The listing builds one solid part. Answer for the finished solid, in the listing's coordinates (mm). A direction names the side the tool comes from. Give positions to 0.01 mm unless a question says otherwise; leave off trailing zeros. Loops run counter-clockwise (first coordinate to the right, second up) from the corner with the lowest first, then second, coordinate; pieces in that order, holes last.
Item 1: Section D-D, the plane y = 31 is taken. Give the vertices of the cut face in (x, z), and give its area (3 significant figures).
Item 2: Section B-B, the plane x = -30 is taken. Give the vertices of the cut face in (y, z).
Item 3: The mould has two halves that part along Z. Classify faces 3 (the face through (75.507, 15.2, 9.693)), 4 (the face through (-1.064, -6.702, 3.125)), 5 (the face through (-76, 15, 20)), 6 (the face through (-60.073, -7.059, 27.407)): pulls with the +Z half, pulls with the -Z half, needs draft (parallel to the pull), parting line crosses it, or undercut.
Item 4: A tool of negligible diameter and unlimited length cuts with its end or side. For faces 1 (the face through (-75.493, 15.2, 9.693)), 2 (the face through (75, 15, 20)), from which of +Z, -Z, +X, -X, +Y, -Y can it reach the whole face along a straight path? Write none if from no direction.
Item 5: Section C-C, the plane y = -3.5 is taken. Give the vertices of the cut face in (x, z).
Item 6: Consider line 1 along X through (y, z) = (30, 21.5); line 2 along Z through (x, y) = (39, 1.5); line 3 along Z through (x, y) = (-33.5, 26). Determine where each line is inside the solid, lowest interval first.
Item 7: Each of these flat-tipped pins is pushed along its axis until it touches: pin 1 Ø12 at (x, z) = (-32.5, 35) entering from -Y; pin 2 Ø1.5 at (x, z) = (-46, 11) entering from -Y; pin 3 Ø6 at (x, z) = (-40, 41.5) entering from +Y. Where does it stop, or does it pass through?
Item 8: Section A-A, the plane y = 8 is taken. Give the vertices of the cut face in (x, z), and give its area (3 significant figures).
Autodesk Fusion 360 part; units mm, degrees
sketch "Sketch1" plane through (0, 0, 0) normal (1, 0, 0) x (0, 1, 0)
  line L0 (0, 0) -> (60, 0)
  line L1 (60, 0) -> (49.9725, 11.9503)
  line L2 (49.9725, 11.9503) -> (9.9318, 49.9475)
  line L3 (49.9725, 11.9503) -> (105.1725, 11.9503) construction
  line L4 (9.9318, 49.9475) -> (-0.0682, 49.9475)
  line L5 (0, 0) -> (-13.5946, 6.3393)
  line L6 (0, 0) -> (15, 0) construction
  line L7 (-13.5946, 6.3393) -> (-0.0682, 49.9475)
  dimension "d15" = 60
  dimension "d16" = 15.6
  dimension "d18" = 136.5
  dimension "d19" = 55.2
  dimension "d24" = 155
  dimension "d25" = 15
extrude "Extrude1" add sketch "Sketch1" along normal mid plane 152
shell "Shell1" thickness 1 removed faces 2 at (25.3333, 23.2787, 37.2817) at (25.3333, 56.6575, 3.9834)
sketch "Sketch3" plane through (0, -14.1952, 4.4031) normal (0, -0.9551, 0.2963) x (1, 0, 0)
  line L0 (-76, 2.0272) -> (76, 2.0272)
  line L1 (76, 2.0272) -> (76, 47.685)
  line L2 (76, 47.685) -> (-76, 47.685)
  line L3 (-76, 47.685) -> (-76, 2.0272)
  line L4 (0, 2.0272) -> (0, 47.685)
  line L5 (-69, 24.0272) -> (-69, 33.0272)
  line L6 (-69, 24.0272) -> (-69, 15.0272)
  line L7 (-69, 33.0272) -> (-51, 33.0272)
  line L8 (-51, 33.0272) -> (-51, 15.0272)
  line L9 (-51, 15.0272) -> (-69, 15.0272)
  line L10 (69, 33.0272) -> (51, 33.0272)
  line L11 (51, 33.0272) -> (51, 15.0272)
  line L12 (51, 15.0272) -> (69, 15.0272)
  line L13 (69, 24.0272) -> (69, 15.0272)
  line L14 (69, 24.0272) -> (69, 33.0272)
extrude "Extrude3" add sketch "Sketch3" along normal blind 28 contours L5 L6 L7 L8 L9 | L10 L11 L12 L13 L14
sketch "Sketch4" plane through (0, -40.9382, 12.6983) normal (0, -0.9551, 0.2963) x (1, 0, 0)
  line L0 (-69, 33.0272) -> (-69, 15.0272)
  line L1 (-69, 15.0272) -> (-51, 15.0272)
  line L2 (-51, 15.0272) -> (-51, 33.0272)
  line L3 (-51, 33.0272) -> (-69, 33.0272)
  line L4 (-54.8, 30.2) -> (-65.2, 30.2)
  line L5 (-65.2, 30.2) -> (-65.2, 17.8)
  line L6 (-65.2, 17.8) -> (-54.8, 17.8)
  line L7 (-54.8, 17.8) -> (-54.8, 30.2)
  line L8 (-54.8, 30.2) -> (-65.2, 17.8) construction
  line L9 (-65.2, 30.2) -> (-54.8, 17.8) construction
  line L10 (54.8, 30.2) -> (65.2, 17.8) construction
  line L11 (65.2, 30.2) -> (54.8, 17.8) construction
  line L12 (65.2, 30.2) -> (65.2, 17.8)
  line L13 (65.2, 17.8) -> (54.8, 17.8)
  line L14 (54.8, 17.8) -> (54.8, 30.2)
  line L15 (54.8, 30.2) -> (65.2, 30.2)
  point P0 (-60, 24)
  point P1 (60, 24)
  dimension "d50" = 10.4
  dimension "d51" = 12.4
extrude "Extrude4" cut sketch "Sketch4" against normal blind 28.2 contours L4 L5 L6 L7 | L12 L13 L14 L15
delete_face "DeleteFace1" 10 faces at (69, -16.8801, 27.2514) (57, -18.6576, 21.5207) (52.2667, -33.2104, 37.6121) (63, -22.2393, 41.4778) (51, -25.7944, 30.0165) (-69, -16.8801, 27.2514) (-57, -18.6576, 21.5207) (-52.2667, -33.2104, 37.6121) (-63, -13.325, 38.7127) (-51, -25.7944, 30.0165)
extrude "Extrude5" add 2 faces at (61.7333, -7.5063, 25.2925) (-58.2667, -7.5063, 25.2925) along direction (0, -0.955108, 0.296257) blind 0.2
sketch "Sketch5" plane through (76, 0, 0) normal (1, 0, 0) x (0, 1, 0)
  line L0 (0, 0) -> (60, 0)
  line L1 (60, 0) -> (49.9725, 11.9503)
  line L2 (49.9725, 11.9503) -> (9.9318, 49.9475)
  line L3 (9.9318, 49.9475) -> (-0.0682, 49.9475)
  line L4 (-0.0682, 49.9475) -> (-13.5946, 6.3393)
  line L5 (-13.5946, 6.3393) -> (0, 0)
  circle A0 centre (14, 12) radius 2.6
  circle A1 centre (8, 34) radius 2.6
  dimension "d58" = 5.2
  dimension "d60" = 5.2
extrude "Extrude6" cut sketch "Sketch5" against normal through all contours A0 | A1
extrude "Extrude2" [suppressed]
equation "bucket_width = 152 mm"
equation "bucket_depth = 60 mm"
equation "bucket_back_height = 50 mm"
equation "wall = 4.5 mm"
equation "side_wall = 5.5 mm"
equation "lip = 7 mm"
equation "pivot_ear_thickness = 6 mm"
equation "pivot_hole = 5 mm"
equation "top_flange = 8 mm"
Worked answers:
1. outline: (-76, 0) - (76, 0) - (76, 29.95) - (75, 29.95) - (75, 1) - (-75, 1) - (-75, 29.95) - (-76, 29.95) - close
1. area: 210 mm2
2. outline: (-13.59, 6.34) - (0, 0) - (60, 0) - (59.16, 1) - (0.22, 1) - (-12.38, 6.88) - (0.67, 48.95) - (10.99, 48.95) - (9.93, 49.95) - (-0.07, 49.95) - close
3. face 3: undercut
3. face 4: pulls with the -Z half
3. face 5: needs draft
3. face 6: pulls with the +Z half
4. face 1: +X, -X
4. face 2: +Y
5. outline: (-76, 1.63) - (76, 1.63) - (76, 38.88) - (-76, 38.88) - close; hole (-75, 2.74) - (75, 2.74) - (75, 35.51) - (-75, 35.51) - close
6. line 1: x = -76 to -75, 75 to 76
6. line 2: z = 0 to 1, 48.95 to 49.95
6. line 3: z = 0 to 1
7. pin 1: stops at y = -6.57
7. pin 2: stops at y = -12.38
7. pin 3: stops at y = -0.71
8. outline: (-76, 0) - (76, 0) - (76, 31.4) - (75, 31.4) - (75, 1) - (-75, 1) - (-75, 31.4) - (-76, 31.4) - close; (-76, 36.6) - (-75, 36.6) - (-75, 48.95) - (75, 48.95) - (75, 36.6) - (76, 36.6) - (76, 49.95) - (-76, 49.95) - close
8. area: 389 mm2
